Can you work these out from the model? Positions are in its coordinate system, mm. A direction names the side the tool comes from. Give positions to 0.01 mm unless a question says otherwise; leave off trailing zeros. Loops run counter-clockwise (first coordinate to the right, second up) from the corner with the lowest first, then second, coordinate; pieces in that order, holes last. Notation, with made-up numbers: M 72.25,-30 L 111.25,-30 A25 ccw 111.25,5 Z; hole C 69.5,12.5 d6. An arc over 180 degrees is marked long. One line per item, written item: value. Start each with the question number.
from build123d import *

# Parameters (mm, degrees)
F1_DEPTH = 6
F2_R     = 7
F3_DEPTH = 6
F4_W     = 12
F4_H     = 25
F5_DEPTH = 6
F6_D     = 13


with BuildPart() as f1:
    # F0 (on Front) → F1 (new body)
    with BuildSketch(Plane.XZ):
        with BuildLine():
            Line((6.5, -32), (12.5, -32))
            Line((12.5, -32), (12.5, 32))
            Line((12.5, 32), (-12.5, 32))
            Line((-12.5, 32), (-12.5, -32))
            Line((-12.5, -32), (-6.5, -32))
            Line((-6.5, -32), (-6.5, -12))
            ThreePointArc((-6.5, -12), (0, -5.5), (6.5, -12))
            Line((6.5, -12), (6.5, -32))
        make_face()
    extrude(amount=F1_DEPTH)

    # F2 (on face) → F3 (join)
    with BuildSketch(Plane.XY.offset(32)):
        with BuildLine():
            Line((-12.5, 0), (12.5, 0))
            Line((12.5, 0), (12.5, 12))
            ThreePointArc((12.5, 12), (0, 24.5), (-12.5, 12))
            Line((-12.5, 12), (-12.5, 0))
        make_face()
        with Locations((0, 12)):
            Circle(F2_R, mode=Mode.SUBTRACT)
    extrude(amount=-F3_DEPTH)

    # F4 (on face) → F5 (join)
    with BuildSketch(Plane(origin=(-12.5, 0, 0), x_dir=(0, -1, 0), z_dir=(-1, 0, 0))):
        with Locations((12, 19.5)):
            Rectangle(F4_W, F4_H)
        with BuildLine():
            ThreePointArc((18, 7), (30.5, 19.5), (18, 32))
            Line((18, 32), (18, 7))
        make_face()
    extrude(amount=-F5_DEPTH)

    # F6 (through all)
    with Locations(Plane(origin=(-12.5, 0, 0), x_dir=(0, -1, 0), z_dir=(-1, 0, 0))):
        with Locations((18, 19.5)):
            Hole(F6_D / 2)


solid = f1.part
Q1. I need wall thicknesses on line 1 along X through (y, z) = (-2, -26); line 2 along Z through (x, y) = (-9.5, 20); line 3 along Y through (x, z) = (-5.5, -1). Which ranges of each line are inside material? Lowest first, please.
Q2. If we section it at D-D, the plane x = -10.25: Write out the boundary of the cut face in (y, z), plus the area to 3 significant figures.
Q3. If we section it at B-B, the plane x = 0: Write out the boundary of the cut face in (y, z).
Q4. If we section it at C-C, the plane y = -3: Write out the boundary of the cut face in (x, z), plus the area to 3 significant figures.
Q5. Which directions (+Z, -Z, +X, -X, +Y, -Y) give clear straight access to the entire face, cutting with the end or side of a thin tool? Please do faces 4 (the face through (0, 0, 4)), 5 (the face through (-6.5, -13, 14)), 6 (the face through (6.5, -3, -22)).
Q6. If we section it at A-A, the plane z = 19.5: Write out the boundary of the cut face in (x, y), plus the area to 3 significant figures.
Q7. If we mould it in two halves opening along Z, with no side actions, what happens to faces 1 (the face through (0, 4, 32)), 2 (the face through (-10, -3, -32)), 3 (the face through (-9.458, -22.791, 23.893))? For each: released by +Z, released by -Z, zero draft, split by the parting line, or undercut.
Q8. For P1, Ø5, axis at x = -8, y = -10, coming from the -Z side; P2, Ø17, axis at y = -18, z = 19.5, coming from the +X side, each with a flat end and sliding along its axis, tell me the tip position at first contact or that it passes through.
Response:
1. line 1: -12.5 to -6.5, 6.5 to 12.5
1. line 2: 26 to 32
1. line 3: -6 to 0
2. outline: M -18,7 L -6,7 L -6,-32 L 0,-32 L 0,26 L 19.15,26 L 19.15,32 L -18,32 A12.5 ccw Z; hole C -18,19.5 d13
2. area: 912 mm^2
3. outline: M -6,-5.5 L 0,-5.5 L 0,26 L 5,26 L 5,32 L -6,32 Z; M 19,26 L 24.5,26 L 24.5,32 L 19,32 Z
4. outline: M -12.5,-32 L -6.5,-32 L -6.5,-12 A6.5 cw 6.5,-12 L 6.5,-32 L 12.5,-32 L 12.5,32 L -12.5,32 Z
4. area: 1,270 mm^2
5. face 4: -Z, +X, -X, +Y
5. face 5: +Z, -Z, +X, -Y
5. face 6: -Z, +Y, -Y
6. outline: M -12.5,-30.5 L -6.5,-30.5 L -6.5,-24.5 L -12.5,-24.5 Z; M -12.5,-11.5 L -6.5,-11.5 L -6.5,-6 L 12.5,-6 L 12.5,0 L -12.5,0 Z
6. area: 219 mm^2
7. face 1: released by +Z
7. face 2: released by -Z
7. face 3: undercut
8. P1: z = 7
8. P2: x = -6.5
